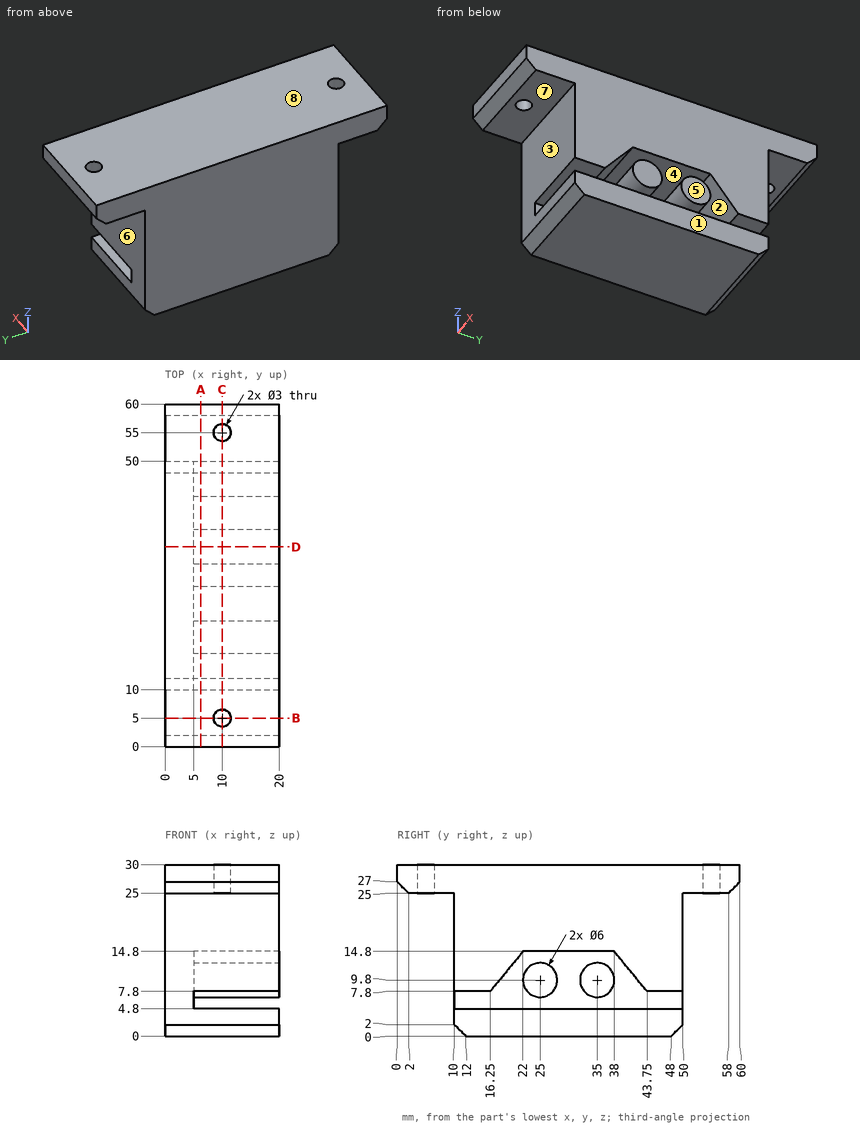
Source: three-view drawing plus pictorial views. Frame: mm from the lowest corner of the part. A direction names the side the tool comes from. Give positions to 0.01 mm unless a question says otherwise; leave off trailing zeros. Order: outer loops, then holes, each group sorted by start corner. A loop starts at its lowest first (then second) coordinate and runs counter-clockwise, first axis right, second up. Notation, with made-up numbers: (27.5, 33.25) - (33.5, 33.25) arc R16 cw to (33.5, 47.25) - close; hole circle Ø4 at (56, 78). An arc over 180 degrees is marked (long way). Answer as a JSON object with one key per item and string values. Group by question number.
Q1. Cut plane D-D, the plane y = 35. Output: boundary loops of the cut face in (x, z).
Q2. Cut plane C-C, the plane x = 10. Count the separate pieces of the cut face and the enclosed holes in it, then the cut area to 3 significant figures.
Q3. Mould query, pull axis Y, two halves, no side actions, for the marked faces 1, 2 and 3. Classes: pulls with the +Y half, pulls with the -Y half, needs draft (parallel to the pull), parting line crosses it, or undercut.
Q4. First-contact query: pin 1 Ø4 at (x, y) = (13.5, 56) entering from -Z; pin 2 Ø5 at (x, z) = (11.5, 7.5) entering from +Y; pin 3 Ø12 at (y, z) = (20.5, 9) entering from +X; pin 4 Ø10 at (x, z) = (14.5, 17.5) entering from -Y. Flat tips, straight axial feed; report the tip coordinate or a pass-through.
Q5. Cut plane B-B, the plane y = 5. Output: boundary loops of the cut face in (x, z).
Q6. Line query: probe 1 along Y at (x, z) = (10, 28.5); probe 2 along Z at (x, y) = (9.5, 35); probe 3 along Z at (x, y) = (16.75, 29.5). Output: solid intervals per line, ascending.
Q7. Set-up query: the marked faces 4, 5, 6, 7 and 8. Return all of +Z, -Z, +X, -X, +Y, -Y with unobstructed straight access to the full face (end or side cutting, diameter ignored); none if empty.
Q8. Cut plane A-A, the plane x = 6.25. Output: boundary loops of the cut face in (y, z).
Results:
{
 "1": {"outline": "(0, 0) - (20, 0) - (20, 4.8) - (5, 4.8) - (5, 6.8) - (20, 6.8) - (20, 12.8) - (5, 12.8) - (5, 14.8) - (20, 14.8) - (20, 30) - (0, 30) - close"},
 "2": {"separate pieces": "6", "enclosed holes": "0", "area": "1,050 mm^2"},
 "3": {"face 1": "needs draft", "face 2": "undercut", "face 3": "pulls with the -Y half"},
 "4": {"pin 1": "z = 25", "pin 2": "y = 50", "pin 3": "x = 20", "pin 4": "y = 10"},
 "5": {"outline": "(0, 25) - (8.5, 25) - (8.5, 30) - (0, 30) - close; (11.5, 25) - (20, 25) - (20, 30) - (11.5, 30) - close"},
 "6": {"probe 1": "0 to 3.5, 6.5 to 53.5, 56.5 to 60", "probe 2": "0 to 4.8, 6.8 to 12.8, 14.8 to 30", "probe 3": "0 to 4.8, 14.8 to 30"},
 "7": {"face 4": "+X", "face 5": "+Z, -Z, +X, +Y, -Y", "face 6": "-Z, +X, -X, +Y", "face 7": "-Z, +X, -X, -Y", "face 8": "+Z, +X, -X, +Y, -Y"},
 "8": {"outline": "(0, 27) - (2, 25) - (10, 25) - (10, 7.8) - (16.25, 7.8) - (22, 14.8) - (38, 14.8) - (43.75, 7.8) - (50, 7.8) - (50, 25) - (58, 25) - (60, 27) - (60, 30) - (0, 30) - close; (10, 2) - (12, 0) - (48, 0) - (50, 2) - (50, 4.8) - (10, 4.8) - close; circle Ø6 at (25, 9.8); circle Ø6 at (35, 9.8)"}
}
